```python
from build123d import *

# Parameters (mm, degrees)
BOSS_EXTRUDE1_DEPTH = 5.08
SKETCH3_R           = 1.5
CUT_EXTRUDE1_DEPTH  = 5.08
CUT_EXTRUDE2_DEPTH  = 7.62
SKETCH5_R           = 1.5
CUT_EXTRUDE3_DEPTH  = 2.54


with BuildPart() as part:
    # Sketch2 → Boss-Extrude1 (new body)
    with BuildSketch(Plane.XY):
        Polygon((-7.754517134, 6.868286604), (11.295482866, 6.868286604), (4.316417445, -18.531713396), (-14.733582555, -18.531713396), align=None)
    extrude(amount=BOSS_EXTRUDE1_DEPTH)

    # Sketch3 → Cut-Extrude1 (cut)
    with BuildSketch(Plane(origin=(0, 6.868286604, 0), x_dir=(1, 0, 0), z_dir=(0, 1, 0))):
        with Locations(Location((6.850482866, -2.54, 0), (0, 0, 270))):
            Circle(SKETCH3_R)
        with Locations(Location((-3.309517134, -2.54, 0), (0, 0, 270))):
            Circle(SKETCH3_R)
    extrude(amount=-CUT_EXTRUDE1_DEPTH, mode=Mode.SUBTRACT)

    # Sketch4 → Cut-Extrude2 (cut)
    with BuildSketch(Plane(origin=(0, 0, 0), x_dir=(-1, 0, 0), z_dir=(0, 0, -1))):
        Polygon((-7.203649611, 5.025464096), (-8.423391825, 2.370731042), (-5.904798927, -6.376274022), (-2.786072566, -6.376274022), (6.889117517, 1.455631702), (3.999397468, 5.025464096), align=None)
        Polygon((8.115115025, 0.956019878), (10.704300182, -10.086093291), (-4.679537518, -11.209249583), (-5.476805356, -7.809136742), (-2.786072566, -7.809136742), align=None)
        Polygon((-4.271117048, -12.434510993), (-3.011820599, -16.961171201), (12.721835887, -16.961171201), (11.237306322, -11.624889252), align=None)
    extrude(amount=-CUT_EXTRUDE2_DEPTH, mode=Mode.SUBTRACT)

    # Sketch5 → Cut-Extrude3 (cut)
    with BuildSketch(Plane.XZ.offset(18.531713396)):
        with Locations(Location((-0.128582555, 2.54, 0), (0, 0, 270))):
            Circle(SKETCH5_R)
        with Locations(Location((-10.288582555, 2.54, 0), (0, 0, 270))):
            Circle(SKETCH5_R)
    extrude(amount=-CUT_EXTRUDE3_DEPTH, mode=Mode.SUBTRACT)


solid = part.part
```
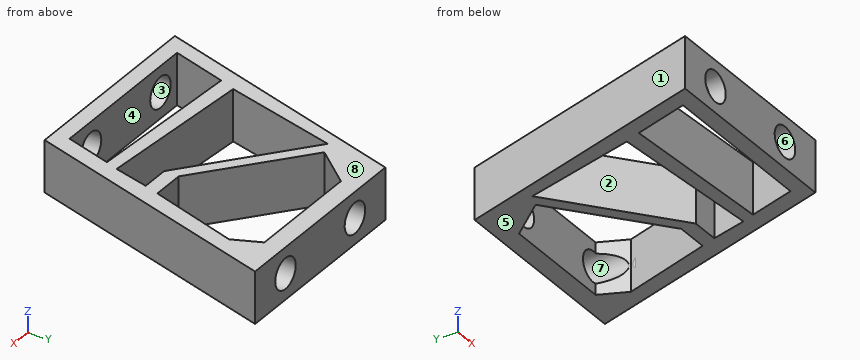
Source: CAD feature listing. Evaluate the final solid. Frame: model axes, mm. Face numbers are marked on the shaded views. A direction names the side the tool comes from. Coordinates: 2 decimals unless noted, no trailing zeros. Loops run counter-clockwise (first coordinate to the right, second up) from the corner with the lowest first, then second, coordinate; pieces in that order, holes last. Notation, with made-up numbers: M -3,49 L 37,49 A24 ccw 37,73 Z; hole C 34.5,63.25 d4. An arc over 180 degrees is marked long. Use a Markdown table: item, result. Add a question column.
Q1. Section query C-C, the plane y = -1. Return loops of the section in (x, z).
Q2. First-contact query: pin 1 (1 mm diameter, centred on y = 2, z = 2.5, fed in from +X). Flat tip, straight axial feed; report the tip coordinate or a pass-through.
Q3. Draft query along Y for the marked faces 1, 2 and 3. Return one class per face: pulls with the +Y half, pulls with the -Y half, needs draft (parallel to the pull), parting line crosses it, or undercut.
Q4. Access query for the marked faces 4, 5, 6, 7 and 8. Directions: +Z, -Z, +X, -X, +Y, -Y. A direction counts if a zero-diameter tool reaches every point of the face in a straight line with its end or side. Return the directions, or none.
Q5. Section query D-D, the plane y = 4.5. Return loops of the section in (x, z).
Q6. Section query B-B, the plane z = 2.54. State how many separate pieces and enclosed holes the cut face has, and give its area (3 significant figures).
Q7. Material intervals for L1, parallel to X at y = -17.9, z = 2.54; L2, parallel to Y at x = 1.75, z = 2.3; L3, parallel to X at y = -4, z = 2.2, sorted ascending.
Q8. Section query A-A, the plane y = -13.5. Return loops of the section in (x, z).
Result:
| question | item | result |
|---|---|---|
| 1 | outline | M -9.92,0 L -8.57,0 L -8.57,5.08 L -9.92,5.08 Z; M -5.68,0 L -3.86,0 L -3.86,5.08 L -5.68,5.08 Z; M 7.45,0 L 9.13,0 L 9.13,5.08 L 7.45,5.08 Z |
| 2 | pin 1 | stops at x = 10.1 |
| 3 | face 1 | pulls with the +Y half |
| 3 | face 2 | undercut |
| 3 | face 3 | needs draft |
| 4 | face 4 | +Z, -Z |
| 4 | face 5 | -Z, +X, -X, +Y, -Y |
| 4 | face 6 | -Y |
| 4 | face 7 | +Y |
| 4 | face 8 | +Z, +X, -X, +Y, -Y |
| 5 | outline | M -8.41,0 L -4.42,0 L -4.42,1.54 A1.5 cw -4.42,3.54 L -4.42,5.08 L -8.41,5.08 Z; M 7.45,0 L 10.64,0 L 10.64,5.08 L 7.45,5.08 L 7.45,3.92 A1.5 cw 7.45,1.16 Z |
| 6 | separate pieces | 3 |
| 6 | enclosed holes | 1 |
| 6 | area | 164 mm2 |
| 7 | L1 | x = -14.56 to -11.79, -8.79 to -1.63, 1.37 to 4.49 |
| 7 | L2 | y = -18.53 to -16.96, -12.3 to -11, -6.98 to -5.54, 5.03 to 6.87 |
| 7 | L3 | x = -10.74 to -9.28, -1.95 to -0.15, 6.59 to 8.31 |
| 8 | outline | M -13.35,0 L -11.76,0 L -11.76,5.08 L -13.35,5.08 Z; M 3.97,0 L 5.7,0 L 5.7,5.08 L 3.97,5.08 Z |
